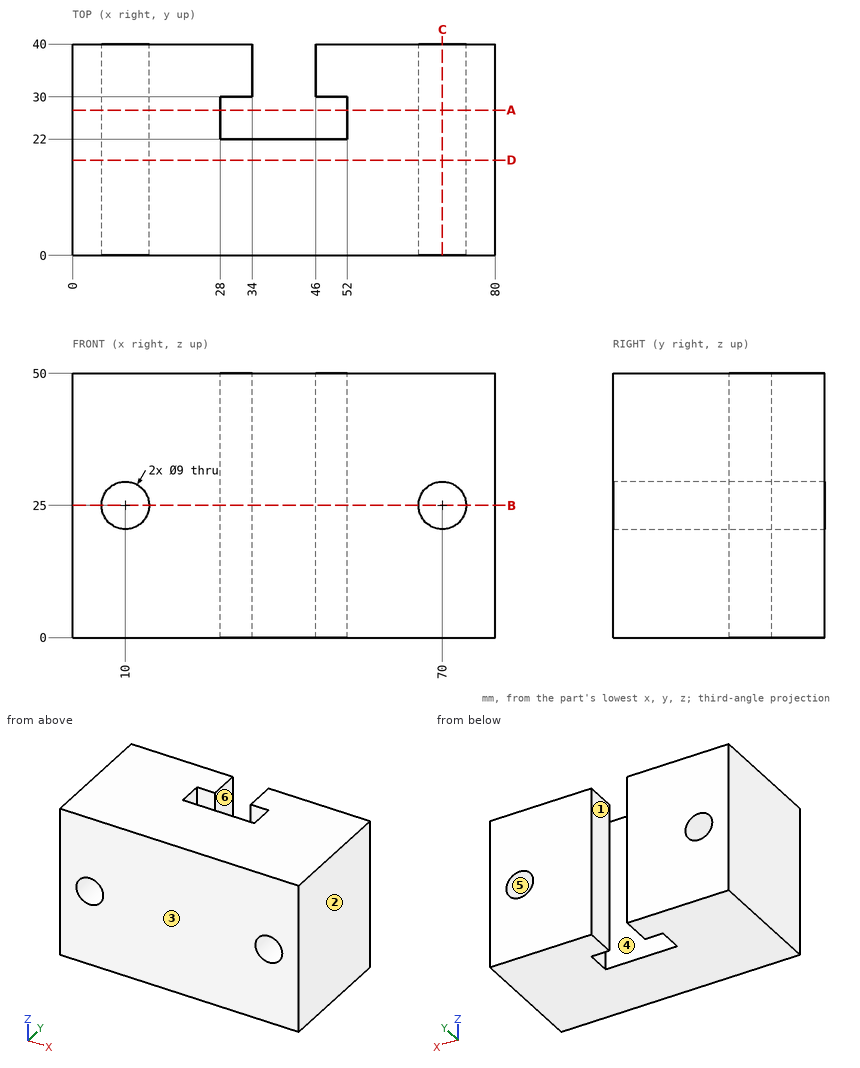
Geometry check sheet. Reference: drawing and pictorial views, mm from the part's lowest x, y, z. A direction names the side the tool comes from. Coordinates: 2 decimals unless noted, no trailing zeros. Write each loop counter-clockwise with the first axis right and the second up, starting at its lowest first coordinate (ties: lowest second). Pieces come first, ordered by that corner, then holes. Notation, with made-up numbers: M 77.25,71.5 L 81.25,71.5 A29 cw 81.25,104.5 Z; hole C -19.5,72.5 d8. An arc over 180 degrees is marked long. Write item = value, one per line. Start each with the question number.
1. Tool access check on the marked faces 4, 5 and 6. Record the directions out of +Z, -Z, +X, -X, +Y, -Y that give a thin tool (end or side, any length) a straight path to the whole face; none if there is none.
2. Sectioned sample at D-D (y = 18). Record the cut outline in (x, z).
3. Sectioned sample at C-C (x = 70). Record the cut outline in (y, z).
4. Sectioned sample at B-B (z = 25). Record the cut outline in (x, y).
5. Thickness scan on probe 1 along X at (y, z) = (27.5, 25); probe 2 along X at (y, z) = (16, 25); probe 3 along Y at (x, z) = (49, 47.5). Record the ranges inside material, lowest first.
6. Sectioned sample at A-A (y = 27.5). Record the cut outline in (x, z), then the cut area to 3 significant figures.
7. Mould release check, pull along X, two halves, no side actions. Record for the marked faces 1, 2 and 3: pulls with the +X half, pulls with the -X half, needs draft (parallel to the pull), parting line crosses it, or undercut.
The answers:
q1.face_4 = +Z, -Z
q1.face_5 = +Y, -Y
q1.face_6 = +Z, -Z, +Y
q2.outline = M 0,0 L 80,0 L 80,50 L 0,50 Z; hole C 10,25 d9; hole C 70,25 d9
q3.outline = M 0,0 L 40,0 L 40,20.5 L 0,20.5 Z; M 0,29.5 L 40,29.5 L 40,50 L 0,50 Z
q4.outline = M 0,0 L 5.5,0 L 5.5,40 L 0,40 Z; M 14.5,0 L 65.5,0 L 65.5,40 L 46,40 L 46,30 L 52,30 L 52,22 L 28,22 L 28,30 L 34,30 L 34,40 L 14.5,40 Z; M 74.5,0 L 80,0 L 80,40 L 74.5,40 Z
q5.probe_1 = 0 to 5.5, 14.5 to 28, 52 to 65.5, 74.5 to 80
q5.probe_2 = 0 to 5.5, 14.5 to 65.5, 74.5 to 80
q5.probe_3 = 0 to 22, 30 to 40
q6.outline = M 0,0 L 28,0 L 28,50 L 0,50 Z; M 52,0 L 80,0 L 80,50 L 52,50 Z; hole C 10,25 d9; hole C 70,25 d9
q6.area = 2,670 mm²
q7.face_1 = undercut
q7.face_2 = pulls with the +X half
q7.face_3 = needs draft
